Could you check a few things on this model? Use its own coordinates, in mm. Face numbers are marked on the shaded views. A direction names the side the tool comes from. Coordinates: 2 decimals unless noted, no trailing zeros. Loops run counter-clockwise (first coordinate to the right, second up) from the corner with the lowest first, then second, coordinate; pieces in that order, holes last. Notation, with made-up numbers: (82, 86) -> (104, 86) arc R18 cw to (104, 120) -> close; hole circle Ø6 at (22, 30.5). An arc over 180 degrees is marked (long way). One line per question, with ' | ' between items. Start each with the question number.
(1) Suppose I cut it at C-C (y = -24). Please give me the cut outline in (x, z), plus the area to 3 significant figures.
(2) If we mould it in two halves opening along X, with no side actions, what happens to the marked faces 3, 4, 5 and 6? For each: pulls with the +X half, pulls with the -X half, needs draft (parallel to the pull), parting line crosses it, or undercut.
(3) I'm going to push flat-ended pins straight in: pin 1 Ø5.5 at (x, z) = (42, 4) entering from -Y; pin 2 Ø10 at (x, y) = (8, 0) entering from +Z; pin 3 Ø0.6 at (x, z) = (47, 9.5) entering from +Y. Where does each tip first touch, or does it pass through?
(4) Which directions (+Z, -Z, +X, -X, +Y, -Y) give clear straight access to the entire face, cutting with the end or side of a thin tool? Please do the marked faces 1 and 2.
(5) If I drill on line 1 along Y through (x, z) = (42, 4.2); line 2 along Y through (x, z) = (-20, 3); line 3 along Y through (x, z) = (35, 6.75), over which ranges is the centre line in solid material (lowest first)?
(6) Suppose I cut it at A-A (x = -35). Give the number of separate pieces and of enclosed holes in the cut face, plus the area to 3 significant figures.
```python
from build123d import *

# Parameters (mm, degrees)
EXTRUDE001_DEPTH  = 2
CYLINDER001_R     = 2.1
CYLINDER001_DEPTH = 11
BOX001_W          = 10
BOX001_H          = 10
BOX001_DEPTH      = 11
FILLET001_R       = 3
CYLINDER_R        = 2
CYLINDER_DEPTH    = 10
BOX_W             = 10
BOX_H             = 80
BOX_DEPTH         = 4
FILLET_R          = 3
SKETCH003_W       = 9.77459
SKETCH003_H       = 44.778202
SKETCH003_W_2     = 16.775318
SKETCH003_H_2     = 11.763574
SKETCH003_W_3     = 22.095015
SKETCH003_H_3     = 27.160165
EXTRUDE003_DEPTH  = 10
EXTRUDE002_DEPTH  = 4
SKETCH_R          = 2.1
EXTRUDE_DEPTH     = 5


with BuildPart() as extrude001:
    # Sketch001 → Extrude001 (new body)
    with BuildSketch(Plane.XY):
        with BuildLine():
            Line((-48, 26.999999), (-48, -26.999999))
            ThreePointArc((-48, -26.999999), (-47.12132, -29.12132), (-44.999999, -30))
            Line((-44.999999, -30), (45.000001, -30))
            ThreePointArc((45.000001, -30), (47.121321, -29.12132), (48, -27))
            Line((48, 27), (48, -27))
            ThreePointArc((48, 27), (47.121321, 29.12132), (45.000001, 30))
            Line((45.000001, 30), (-44.999999, 30))
            ThreePointArc((-44.999999, 30), (-47.12132, 29.12132), (-48, 26.999999))
        make_face()
    extrude(amount=EXTRUDE001_DEPTH)


with BuildPart() as insert_hole:
    # Cylinder001 → Cylinder001 (new body)
    with BuildSketch(Plane.XY):
        Circle(CYLINDER001_R)
    extrude(amount=CYLINDER001_DEPTH)


with BuildPart() as compound:
    # Box001 → Box001 (new body)
    with BuildSketch(Plane(origin=(-5, -5, 0), x_dir=(1, 0, 0), z_dir=(0, 0, 1))):
        with Locations((5, 5)):
            Rectangle(BOX001_W, BOX001_H)
    extrude(amount=BOX001_DEPTH)

    # Fillet001
    fillet001_edges = [compound.edges().sort_by_distance(p)[0] for p in [
        (-5, 5, 5.5),
        (5, 5, 5.5),
    ]]
    fillet(fillet001_edges, radius=FILLET001_R)

    # Cut001: cut insert hole
    add(insert_hole.part, mode=Mode.SUBTRACT)


with BuildPart() as compound_1:
    # Compound placement: moved
    add(compound.part.moved(Location((0, 35, 0))))


with BuildPart() as fusion001:
    # Part__Mirroring002: instance of Compound
    add(compound_1.part.mirror(Plane(origin=(0, 0, 0), x_dir=(1, 0, 0), z_dir=(0, 1, 0))))

    # Fusion001: union Compound
    add(compound_1.part)


with BuildPart() as fusion001_1:
    # Fusion001 placement: moved
    add(fusion001.part.moved(Location((35, 0, 0))))


with BuildPart() as part_mirroring003:
    # Part__Mirroring003: instance of Fusion001
    add(fusion001_1.part.mirror(Plane(origin=(0, 0, 0), x_dir=(0, -1, 0), z_dir=(1, 0, 0))))


with BuildPart() as insert_hole_fusion:
    # Fusion002 base: copy of Fusion001
    add(fusion001_1.part)

    # Fusion002: union Part__Mirroring003
    add(part_mirroring003.part)


with BuildPart() as bolt_hole:
    # Cylinder → Cylinder (new body)
    with BuildSketch(Plane(origin=(0, 35, 0), x_dir=(1, 0, 0), z_dir=(0, 0, 1))):
        Circle(CYLINDER_R)
    extrude(amount=CYLINDER_DEPTH)


with BuildPart() as hole_fusion:
    # Part__Mirroring: instance of bolt hole
    add(bolt_hole.part.mirror(Plane(origin=(0, 0, 0), x_dir=(1, 0, 0), z_dir=(0, 1, 0))))

    # Fusion: union bolt hole
    add(bolt_hole.part)


with BuildPart() as bolt_plate_cut:
    # Box → Box (new body)
    with BuildSketch(Plane(origin=(-5, -40, 0), x_dir=(1, 0, 0), z_dir=(0, 0, 1))):
        with Locations((5, 40)):
            Rectangle(BOX_W, BOX_H)
    extrude(amount=BOX_DEPTH)

    # Fillet
    fillet_edges = [bolt_plate_cut.edges().sort_by_distance(p)[0] for p in [
        (-5, -40, 2),
        (-5, 40, 2),
        (5, -40, 2),
        (5, 40, 2),
    ]]
    fillet(fillet_edges, radius=FILLET_R)

    # Cut: cut hole fusion
    add(hole_fusion.part, mode=Mode.SUBTRACT)


with BuildPart() as bolt_plate_cut_1:
    # Cut placement: moved
    add(bolt_plate_cut.part.moved(Location((20, 0, 0))))


with BuildPart() as part_mirroring001:
    # Part__Mirroring001: instance of bolt plate cut
    add(bolt_plate_cut_1.part.mirror(Plane(origin=(0, 0, 0), x_dir=(0, -1, 0), z_dir=(1, 0, 0))))


with BuildPart() as obj1:
    # Fusion003 base: copy of bolt plate cut
    add(bolt_plate_cut_1.part)

    # Fusion003: union Part__Mirroring001
    add(part_mirroring001.part)


with BuildPart() as holes_extrude003:
    # Sketch003 → Extrude003 (new body)
    with BuildSketch(Plane.XY):
        with Locations((46.967045, 0.099766)):
            Rectangle(SKETCH003_W, SKETCH003_H)
        with Locations((-43.662671, 16.078721)):
            Rectangle(SKETCH003_W_2, SKETCH003_H_2)
        with Locations((-42.010708, -8.32763)):
            Rectangle(SKETCH003_W_3, SKETCH003_H_3)
    extrude(amount=EXTRUDE003_DEPTH)


with BuildPart() as holes_extrude003_1:
    # Extrude003 placement: moved
    add(holes_extrude003.part.moved(Location((0, 0, 7))))


with BuildPart() as cut002:
    # Sketch002 → Extrude002 (new body)
    with BuildSketch(Plane.XY):
        with BuildLine():
            Line((-47.999997, 26.99601), (-48, -27))
            ThreePointArc((-48, -27), (-47.116017, -29.126611), (-44.985018, -29.999963))
            Line((-44.985018, -29.999963), (45.000001, -30))
            ThreePointArc((45.000001, -30), (47.121321, -29.12132), (48, -27))
            Line((48, 27), (48, -27))
            ThreePointArc((48, 27), (47.121321, 29.12132), (45.000001, 30))
            Line((45.000001, 30), (-45, 30))
            ThreePointArc((-45, 30), (-47.122731, 29.119909), (-47.999997, 26.99601))
        make_face()
        with BuildLine():
            Line((-45.2, -28), (45.2, -28))
            ThreePointArc((45.2, -28), (45.765689, -27.765682), (46, -27.199989))
            Line((46, -27.199989), (46, 27.2))
            ThreePointArc((46, 27.2), (45.765685, 27.765685), (45.2, 28))
            Line((45.2, 28), (-45.2, 28))
            ThreePointArc((-45.2, 28), (-45.765685, 27.765685), (-46, 27.2))
            Line((-46, 27.2), (-46, -27.2))
            ThreePointArc((-46, -27.2), (-45.765685, -27.765685), (-45.2, -28))
        make_face(mode=Mode.SUBTRACT)
    extrude(amount=EXTRUDE002_DEPTH)


with BuildPart() as cut002_1:
    # Extrude002 placement: moved
    add(cut002.part.moved(Location((0, 0, 7))))

    # Cut002: cut holes Extrude003
    add(holes_extrude003_1.part, mode=Mode.SUBTRACT)


with BuildPart() as bottom_part:
    # Sketch → Extrude (new body)
    with BuildSketch(Plane.XY):
        with BuildLine():
            Line((-45, 30), (45, 30))
            ThreePointArc((48, 27), (47.12132, 29.12132), (45, 30))
            Line((48, 27), (48, -27))
            ThreePointArc((45, -30), (47.12132, -29.12132), (48, -27))
            Line((45, -30), (-45, -30))
            ThreePointArc((-48, -27), (-47.12132, -29.12132), (-45, -30))
            Line((-48, -27), (-48, 27))
            ThreePointArc((-45, 30), (-47.12132, 29.12132), (-48, 27))
        make_face()
        with Locations((-42, 24)):
            Circle(SKETCH_R, mode=Mode.SUBTRACT)
        with Locations((42, 24)):
            Circle(SKETCH_R, mode=Mode.SUBTRACT)
        with Locations((42, -24)):
            Circle(SKETCH_R, mode=Mode.SUBTRACT)
        with Locations((-42, -24)):
            Circle(SKETCH_R, mode=Mode.SUBTRACT)
        with BuildLine():
            ThreePointArc((-46, 21), (-38.464466, 20.464466), (-39, 28))
            Line((-39, 28), (39, 28))
            ThreePointArc((39, 28), (38.464466, 20.464466), (46, 21))
            Line((46, 21), (46, -21))
            ThreePointArc((46, -21), (38.464466, -20.464466), (39, -28))
            Line((39, -28), (-39, -28))
            ThreePointArc((-39, -28), (-38.464466, -20.464466), (-46, -21))
            Line((-46, -21), (-46, 21))
        make_face(mode=Mode.SUBTRACT)
    extrude(amount=EXTRUDE_DEPTH)


with BuildPart() as bottom_part_1:
    # Extrude placement: moved
    add(bottom_part.part.moved(Location((0, 0, 2))))

    # Fusion004: union Extrude001, insert hole fusion, obj1, Cut002
    add(extrude001.part)
    add(insert_hole_fusion.part)
    add(obj1.part)
    add(cut002_1.part)


solid = bottom_part_1.part
```
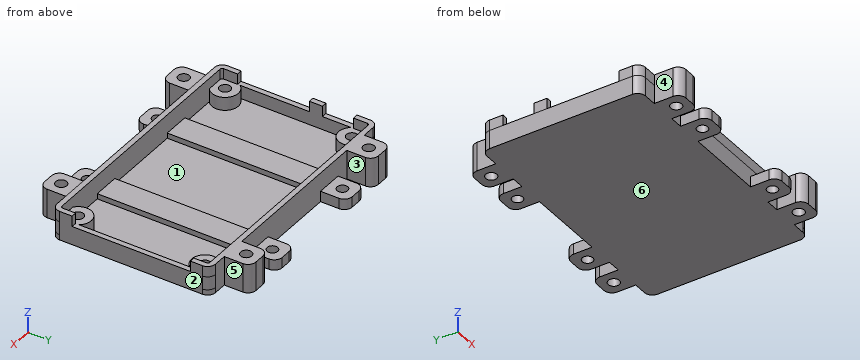
Checks:
1) outline: (-48, 0) -> (48, 0) -> (48, 11) -> (46, 11) -> (46, 7) -> (44.1, 7) -> (44.1, 2) -> (39.9, 2) -> (39.9, 7) -> (37, 7) -> (37, 2) -> (25, 2) -> (25, 4) -> (15, 4) -> (15, 2) -> (-15, 2) -> (-15, 4) -> (-25, 4) -> (-25, 2) -> (-37, 2) -> (-37, 7) -> (-39.9, 7) -> (-39.9, 2) -> (-44.1, 2) -> (-44.1, 7) -> (-46, 7) -> (-46, 11) -> (-48, 11) -> close | area: 316 mm^2
2) face 3: undercut | face 4: pulls with the -X half | face 5: pulls with the +X half | face 6: needs draft
3) pin 1: stops at y = -38.98 | pin 2: stops at z = 2 | pin 3: stops at y = 29.47
4) face 1: +Z | face 2: +Z, -Z, +X, +Y, -Y
5) line 1: y = -30 to -26.1, -21.9 to -19, 19 to 21.9, 26.1 to 30 | line 2: y = -40 to -37, -33 to 33, 37 to 40 | line 3: y = -40 to -37.1, -32.9 to -28, 28 to 32.9, 37.1 to 40
6) separate pieces: 3 | enclosed holes: 0 | area: 284 mm^2
